For this review, take the finished solid that the model builds, in its own axes (mm). A direction names the side the tool comes from. Give positions to 0.01 mm unless a question says otherwise; leave off trailing zeros. Loops run counter-clockwise (first coordinate to the right, second up) from the corner with the lowest first, then second, coordinate; pieces in that order, holes last. Notation, with made-up numbers: (35.25, 34.25) - (46.25, 34.25) arc R9 ccw to (46.25, 43.25) - close; hole circle Ø5 at (81, 4). An arc over 180 degrees is marked (long way). Answer as CSV lines item,"result".
Autodesk Inventor part; units mm, degrees
ref_plane "YZ Plane" through (0, 0, 0) normal (1, 0, 0) x (0, 1, 0)
ref_plane "XZ Plane" through (0, 0, 0) normal (0, 1, 0) x (-1, 0, 0)
ref_plane "XY Plane" through (0, 0, 0) normal (0, 0, 1) x (1, 0, 0)
sketch "Sketch1" plane through (0, 0, 0) normal (0, 0, 1) x (1, 0, 0)
  line L0 (-15, 15) -> (15, 15)
  line L1 (15, 15) -> (15, -15)
  line L2 (15, -15) -> (-15, -15)
  line L3 (-15, -15) -> (-15, 15)
  point P0 (0, 0)
  dimension "d0" = 30
  dimension "d1" = 30
  dimension "d2" = 15
  dimension "d3" = 15
extrude "Extrusion1" add sketch "Sketch1" along normal blind 12
sketch "Sketch2" plane through (0, 0, 12) normal (0, 0, 1) x (1, 0, 0)
  circle A0 centre (0, 5) radius 2.25
  line L0 (15, 15) -> (-15, 15)
  dimension "d34" = 4.5
  dimension "d35" = 10
extrude "Extrusion2" cut sketch "Sketch2" against normal blind 12
sketch "Sketch3" plane through (0, 0, 12) normal (0, 0, 1) x (1, 0, 0)
  circle A0 centre (0, 5) radius 4.25
  line L0 (15, 15) -> (-15, 15)
  dimension "d32" = 8.5
  dimension "d33" = 10
extrude "Extrusion3" cut sketch "Sketch3" against normal blind 5.5
sketch "Sketch4" plane through (0, 0, 12) normal (0, 0, 1) x (1, 0, 0)
  line L0 (0, 0) -> (0, 18.2)
  line L1 (0, 18.2) -> (-18.0312, 0.1688)
  line L2 (0, 18.2) -> (18.0312, 0.1688)
  line L3 (0, 18.2) -> (25.5, 18.2) construction
  line L4 (18.0312, 0.1688) -> (-18.0312, 0.1688)
  dimension "d12" = 18.2
  dimension "d13" = 25.5
  dimension "d14" = 45
  dimension "d26" = 25.5
  dimension "d27" = 45
extrude "Extrusion4" cut sketch "Sketch4" against normal blind 1
sketch "Sketch5" plane through (0, 0, 12) normal (0, 0, 1) x (1, 0, 0)
  circle A0 centre (10, -10) radius 2.25
  line L0 (-15, -15) -> (15, -15)
  line L1 (15, -15) -> (15, 15)
  circle A1 centre (-10, -10) radius 2.25
  line L2 (-15, 0.1688) -> (-15, -15)
  point P0 (0, 0)
  point P1 (15, 0.3223)
  point P2 (-15, 0.3223)
  dimension "d18" = 4.5
  dimension "d19" = 5
  dimension "d20" = 5
  dimension "d21" = 4.5
  dimension "d22" = 5
  dimension "d23" = 5
extrude "Extrusion5" cut sketch "Sketch5" against normal blind 12
sketch "Sketch6" plane through (0, 0, 12) normal (0, 0, 1) x (1, 0, 0)
  circle A0 centre (-10, -10) radius 2.25
  line L0 (-12.1651, -13.75) -> (-14.3301, -10)
  line L1 (-14.3301, -10) -> (-12.1651, -6.25)
  line L2 (-12.1651, -6.25) -> (-7.8349, -6.25)
  line L3 (-7.8349, -6.25) -> (-5.6699, -10)
  line L4 (-5.6699, -10) -> (-7.8349, -13.75)
  line L5 (-7.8349, -13.75) -> (-12.1651, -13.75)
  circle A1 centre (10, -10) radius 2.25
  line L6 (7.8349, -13.75) -> (5.6699, -10)
  line L7 (5.6699, -10) -> (7.8349, -6.25)
  line L8 (7.8349, -6.25) -> (12.1651, -6.25)
  line L9 (12.1651, -6.25) -> (14.3301, -10)
  line L10 (14.3301, -10) -> (12.1651, -13.75)
  line L11 (12.1651, -13.75) -> (7.8349, -13.75)
  point P0 (0, 0)
  dimension "d28" = 7.5
  dimension "d29" = 7.5
extrude "Extrusion6" cut sketch "Sketch6" against normal blind 4
properties part number "210505 - Prism adapter v3"
1) Consider section D-D on y = 1.25. Write out the cut boundary in (x, z).
From the geometry:
outline,"(-15, 0) - (15, 0) - (15, 11) - (2, 11) - (2, 6.5) - (-2, 6.5) - (-2, 11) - (-15, 11) - close"
2) Wall thickness on line 1 (Y direction, x = 10, z = 4.25); line 2 (Y direction, x = 0, z = 4.25); line 3 (X direction, y = -11.75, z = 5.75): over which ranges is each line inside the solid? List them lowest first. Write a range as from..to.
From the geometry:
line 1,"y = -15..-12.25, -7.75..15"
line 2,"y = -15..2.75, 7.25..15"
line 3,"x = -15..-11.41, -8.59..8.59, 11.41..15"
3) Consider section C-C on z = 2. Write out the cut boundary in (x, y).
From the geometry:
outline,"(-15, -15) - (15, -15) - (15, 15) - (-15, 15) - close; hole circle Ø4.5 at (-10, -10); hole circle Ø4.5 at (0, 5); hole circle Ø4.5 at (10, -10)"
4) Draft analysis for pull direction X (two halves, no side actions). For faces 4 (the flat face through (15, 0, 6)), 5 (the flat face through (0, -15, 6)), 6 (the flat face through (-13.26, -8.15, 10.03)), state which applies: pulls with the +X half, pulls with the -X half, needs draft (parallel to the pull), parting line crosses it, or undercut.
From the geometry:
face 4,"pulls with the +X half"
face 5,"needs draft"
face 6,"undercut"
5) Consider section A-A on y = 5. Write out the cut boundary in (x, z).
From the geometry:
outline,"(-15, 0) - (-2.25, 0) - (-2.25, 6.5) - (-4.25, 6.5) - (-4.25, 11) - (-13.2, 11) - (-13.2, 12) - (-15, 12) - close; (2.25, 0) - (15, 0) - (15, 12) - (13.2, 12) - (13.2, 11) - (4.25, 11) - (4.25, 6.5) - (2.25, 6.5) - close"
6) Insertion check: P1, Ø4, axis at x = 9, y = -8.5, coming from the +Z side; P2, Ø2.5, axis at x = -1, y = 3, coming from the +Z side. Each pin has a flat end and moves straight along its axis. Give the tip position at first contact, or say it passes through.
From the geometry:
P1,"stops at z = 8"
P2,"stops at z = 6.5"
7) Machinability: for faces 1 (the cylindrical face through (8.34, -8.48, 4.06)), 2 (the flat face through (-10, -6.25, 10)), 3 (the flat face through (0.2, 0.169, 11.5)), which of the approach directions +Z, -Z, +X, -X, +Y, -Y give a long, thin tool a straight path to every point of the face, cutting with its end or side? Answer none if there is none.
From the geometry:
face 1,"+Z, -Z"
face 2,"+Z"
face 3,"+Z, +X, -X"
8) Consider section B-B on x = -10. Write out the cut boundary in (y, z).
From the geometry:
outline,"(-15, 0) - (-12.25, 0) - (-12.25, 8) - (-13.75, 8) - (-13.75, 12) - (-15, 12) - close; (-7.75, 0) - (15, 0) - (15, 12) - (8.2, 12) - (8.2, 11) - (0.17, 11) - (0.17, 12) - (-6.25, 12) - (-6.25, 8) - (-7.75, 8) - close"
